from build123d import *

# Parameters (mm, degrees)
SKETCH_1_W       = 300
SKETCH_1_H       = 250
EXTRUDE_1_DEPTH  = 25
SKETCH_2_W       = 20
SKETCH_2_H       = 20
EXTRUDE_3_DEPTH  = 200
SKETCH_3_W       = 20
SKETCH_3_H       = 20
EXTRUDE_4_DEPTH  = 20
SKETCH_4_W       = 20
SKETCH_4_H       = 20
EXTRUDE_5_DEPTH  = 20
SKETCH_5_W       = 20
SKETCH_5_H       = 20
EXTRUDE_6_DEPTH  = 20
SKETCH_6_W       = 20
SKETCH_6_H       = 20
EXTRUDE_7_DEPTH  = 20
EXTRUDE_8_REACH  = 450.247
SKETCH_8_W       = 20
SKETCH_8_H       = 20
EXTRUDE_9_REACH  = 452.472
SKETCH_9_W       = 20
SKETCH_9_H       = 20
SKETCH_10_W      = 300
SKETCH_10_H      = 10
EXTRUDE_11_DEPTH = 20


with BuildPart() as part:
    # 草图1 → 凸台-拉伸1 (new body)
    with BuildSketch(Plane.XY):
        with Locations((150, 125)):
            Rectangle(SKETCH_1_W, SKETCH_1_H)
    extrude(amount=EXTRUDE_1_DEPTH)

    # 草图2 → 凸台-拉伸3 (add)
    with BuildSketch(Plane.XY.offset(25)):
        with Locations((10, 10)):
            Rectangle(SKETCH_2_W, SKETCH_2_H)
        with Locations((10, 240)):
            Rectangle(SKETCH_2_W, SKETCH_2_H)
        with Locations((290, 240)):
            Rectangle(SKETCH_2_W, SKETCH_2_H)
        with Locations((290, 10)):
            Rectangle(SKETCH_2_W, SKETCH_2_H)
    extrude(amount=EXTRUDE_3_DEPTH)

    # 草图3 → 凸台-拉伸4 (add)
    with BuildSketch(Plane.XY.offset(225)):
        with Locations((10, 10)):
            Rectangle(SKETCH_3_W, SKETCH_3_H)
    extrude(amount=EXTRUDE_4_DEPTH)

    # 草图4 → 凸台-拉伸5 (add)
    with BuildSketch(Plane.XY.offset(225)):
        with Locations((290, 10)):
            Rectangle(SKETCH_4_W, SKETCH_4_H)
    extrude(amount=EXTRUDE_5_DEPTH)

    # 草图5 → 凸台-拉伸6 (add)
    with BuildSketch(Plane.XY.offset(225)):
        with Locations((290, 240)):
            Rectangle(SKETCH_5_W, SKETCH_5_H)
    extrude(amount=EXTRUDE_6_DEPTH)

    # 草图6 → 凸台-拉伸7 (add)
    with BuildSketch(Plane.XY.offset(225)):
        with Locations((10, 240)):
            Rectangle(SKETCH_6_W, SKETCH_6_H)
    extrude(amount=EXTRUDE_7_DEPTH)

    # 草图8 → 凸台-拉伸8 (add, up to next)
    with BuildSketch(Plane(origin=(20, 0, 0), x_dir=(0, 0, -1), z_dir=(1, 0, 0)), mode=Mode.PRIVATE) as extrude_8_sk1:
        with Locations((-235, 10)):
            Rectangle(SKETCH_8_W, SKETCH_8_H)
    extrude_8_tool1 = extrude(extrude_8_sk1.sketch, amount=EXTRUDE_8_REACH, mode=Mode.PRIVATE) - part.part
    # 草图8 → 凸台-拉伸8 (add, up to next)
    with BuildSketch(Plane(origin=(20, 0, 0), x_dir=(0, 0, -1), z_dir=(1, 0, 0)), mode=Mode.PRIVATE) as extrude_8_sk2:
        with Locations((-235, 240)):
            Rectangle(SKETCH_8_W, SKETCH_8_H)
    extrude_8_tool2 = extrude(extrude_8_sk2.sketch, amount=EXTRUDE_8_REACH, mode=Mode.PRIVATE) - part.part
    add(extrude_8_tool1.solids().sort_by_distance((20, 10, 235))[0])
    add(extrude_8_tool2.solids().sort_by_distance((20, 240, 235))[0])

    # 草图9 → 凸台-拉伸9 (add, up to next)
    with BuildSketch(Plane(origin=(0, 230, 0), x_dir=(-1, 0, 0), z_dir=(0, -1, 0)), mode=Mode.PRIVATE) as extrude_9_sk1:
        with Locations((-10, -215)):
            Rectangle(SKETCH_9_W, SKETCH_9_H)
    extrude_9_tool1 = extrude(extrude_9_sk1.sketch, amount=EXTRUDE_9_REACH, mode=Mode.PRIVATE) - part.part
    # 草图9 → 凸台-拉伸9 (add, up to next)
    with BuildSketch(Plane(origin=(0, 230, 0), x_dir=(-1, 0, 0), z_dir=(0, -1, 0)), mode=Mode.PRIVATE) as extrude_9_sk2:
        with Locations((-290, -215)):
            Rectangle(SKETCH_9_W, SKETCH_9_H)
    extrude_9_tool2 = extrude(extrude_9_sk2.sketch, amount=EXTRUDE_9_REACH, mode=Mode.PRIVATE) - part.part
    add(extrude_9_tool1.solids().sort_by_distance((10, 230, 215))[0])
    add(extrude_9_tool2.solids().sort_by_distance((290, 230, 215))[0])

    # 草图10 → 凸台-拉伸11 (add)
    with BuildSketch(Plane.XY.offset(245)):
        with Locations((150, 245)):
            Rectangle(SKETCH_10_W, SKETCH_10_H)
        with Locations((150, 5)):
            Rectangle(SKETCH_10_W, SKETCH_10_H)
    extrude(amount=EXTRUDE_11_DEPTH)


solid = part.part
CAD build for the part. Positions are in the model's coordinates, mm. A direction names the side the tool comes from. Coordinates: 2 decimals unless noted, no trailing zeros. Write each loop counter-clockwise with the first axis right and the second up, starting at its lowest first coordinate (ties: lowest second). Pieces come first, ordered by that corner, then holes. Notation, with made-up numbers: M 36,39.25 L 86,39.25 A28 ccw 86,70.25 Z; hole C 53,89.5 d3. An arc over 180 degrees is marked long. Return JSON: item names as keys, results as strings.
Item 1: Slice it at C-C, the plane y = 111. Write the cut outline in (x, z), and give its area (3 significant figures).
Findings below:
{"outline": "M 0,0 L 300,0 L 300,25 L 0,25 Z; M 0,205 L 20,205 L 20,225 L 0,225 Z; M 280,205 L 300,205 L 300,225 L 280,225 Z", "area": "8,300 mm2"}
Item 2: Slice it at A-A, the plane x = 147. Write the cut outline in (y, z).
Findings below:
{"outline": "M 0,0 L 250,0 L 250,25 L 0,25 Z; M 0,225 L 20,225 L 20,245 L 10,245 L 10,265 L 0,265 Z; M 230,225 L 250,225 L 250,265 L 240,265 L 240,245 L 230,245 Z"}
Item 3: Probe line 1 (Y direction, x = 122.5, z = 235); line 2 (X direction, y = 11, z = 156.5); line 3 (Z direction, x = 108.5, y = 184). List the from-to ranges inside material, lowest first. Write a range as from..to.
Findings below:
{"line 1": "y = 0..20, 230..250", "line 2": "x = 0..20, 280..300", "line 3": "z = 0..25"}
Item 4: Slice it at B-B, the plane z = 112.5. Write the cut outline in (x, y).
Findings below:
{"outline": "M 0,0 L 20,0 L 20,20 L 0,20 Z; M 0,230 L 20,230 L 20,250 L 0,250 Z; M 280,0 L 300,0 L 300,20 L 280,20 Z; M 280,230 L 300,230 L 300,250 L 280,250 Z"}
Item 5: Which spindle directions (+Z, -Z, +X, -X, +Y, -Y) get a long thin tool onto all of the face, cutting with end or side? Do faces 4 (the flat face through (148, 235, 245)), 5 (the flat face through (10, 20, 116)), 6 (the flat face through (20, 126, 207)). Say none if no direction does.
Findings below:
{"face 4": "+Z, +X, -X", "face 5": "+X, -X", "face 6": "+Y, -Y"}
Item 6: Two-plate mould, pull along Y, no slides. Class faces 1 (the flat face through (280, 126, 207)), 2 (the flat face through (290, 230, 116)), 3 (the flat face through (290, 126, 225)): +Y half, -Y half, draft (parallel to the pull), parting line (faces both ways), or undercut.
Findings below:
{"face 1": "draft", "face 2": "undercut", "face 3": "undercut"}
Item 7: Drop flat-ended pins along their axis: pin 1 Ø2 at (x, y) = (189.5, 47.5) entering from +Z; pin 2 Ø4 at (x, y) = (60, 50) entering from -Z; pin 3 Ø12 at (y, z) = (103.5, 36) entering from +X; pin 4 Ø6 at (x, y) = (10.5, 118.5) entering from +Z. Give the stop position or say it passes through.
Findings below:
{"pin 1": "stops at z = 25", "pin 2": "stops at z = 0", "pin 3": "passes through", "pin 4": "stops at z = 225"}
